Part model, mm, in its own coordinate system. Face numbers are marked on the shaded views. A direction names the side the tool comes from. Give positions to 0.01 mm unless a question says otherwise; leave off trailing zeros. Order: outer loops, then holes, each group sorted by start corner. A loop starts at its lowest first (then second) coordinate and runs counter-clockwise, first axis right, second up. Notation, with made-up numbers: (75, 21.25) - (114, 21.25) arc R11 cw to (114, 37.25) - close; hole circle Ø4 at (-21.5, 58). An arc over 180 degrees is marked (long way). One line per item, written item: value.
Autodesk Inventor part; units mm, degrees
ref_plane "YZ Plane" through (0, 0, 0) normal (1, 0, 0) x (0, 1, 0)
ref_plane "XZ Plane" through (0, 0, 0) normal (0, 1, 0) x (-1, 0, 0)
ref_plane "XY Plane" through (0, 0, 0) normal (0, 0, 1) x (1, 0, 0)
sketch "Эскиз1" plane through (0, 0, 0) normal (0, 0, 1) x (1, 0, 0)
  line L0 (-15, -15) -> (15, -15)
  line L1 (15, -15) -> (15, 15)
  line L2 (15, 15) -> (-15, 15)
  line L3 (-15, 15) -> (-15, -15)
  line L4 (-15, -15) -> (15, 15) construction
  line L5 (15, -15) -> (-15, 15) construction
  line L6 (15, 15) -> (20, 15)
  line L7 (20, 15) -> (20, -15)
  line L8 (20, -15) -> (15, -15)
  line L9 (15, -15) -> (15, 15)
  point P0 (0, 0)
  dimension "d0" = 30
  dimension "d1" = 30
  dimension "d2" = 5
extrude "Выдавливание1" add sketch "Эскиз1" along normal blind 5
sketch "Эскиз2" plane through (0, 0, 0) normal (0, 0, -1) x (-1, 0, 0)
  line L0 (-20, -15) -> (-20, 15)
  line L1 (15, -15) -> (-20, -15)
  line L2 (-20, 15) -> (-15, 15)
  line L3 (-15, 15) -> (-15, -15)
  line L4 (-15, -15) -> (-20, -15)
  line L5 (-20, -15) -> (-20, 15)
  point P0 (0, 0)
  dimension "d7" = 5
extrude "Выдавливание2" add sketch "Эскиз2" along normal blind 30
sketch "Эскиз3" plane through (0, 0, 5) normal (0, 0, 1) x (1, 0, 0)
  line L0 (-15, 15) -> (-15, -15)
  line L1 (-15, 0) -> (0, 0)
  circle A0 centre (0, 0) radius 4.1
  dimension "d10" = 15
  dimension "d11" = 8.2
sketch "Эскиз4" plane through (20, -15, 5) normal (1, 0, 0) x (0, 0, -1)
  line L0 (35, 30) -> (35, 0)
  line L1 (35, 15) -> (20, 15)
  circle A0 centre (20, 15) radius 4.1
  point P0 (5, 15)
  dimension "d12" = 15
  dimension "d13" = 8.2
sketch "Эскиз5" plane through (-15, 15, 5) normal (0, 1, 0) x (1, 0, 0)
  line L0 (30, 5) -> (30, 35)
  line L1 (30, 5) -> (50, 5)
  line L2 (50, 5) -> (50, -15)
  line L3 (50, -15) -> (30, -15)
  line L4 (30, -15) -> (30, 5)
  point P0 (15, 5)
  dimension "d18" = 20
  dimension "d19" = 20
extrude "Выдавливание5" add sketch "Эскиз5" against normal blind 5
chamfer "Фаска1" distance 15 angle 45 2 edges at (20, 12.5, 0) (15, 12.5, 5)
chamfer "Фаска2" distance 10 angle 45 2 edges at (17.5, 10, 5) (20, 10, 2.5)
extrude "Выдавливание6" cut sketch "Эскиз3" along normal blind 5 and the other way blind 16.25
extrude "Выдавливание7" cut sketch "Эскиз4" along normal blind 5 and the other way blind 11.5
sketch "Эскиз6" plane through (0, 0, 5) normal (0, 0, 1) x (1, 0, 0)
  circle A0 centre (0, 0) radius 7.5
  dimension "d38" = 15
extrude "Выдавливание8" cut sketch "Эскиз6" along normal blind 10.5
sketch "Эскиз7" plane through (20, -15, -30) normal (1, 0, 0) x (0, 0, -1)
  arc A0 (-19.1, 15) -> (-15, 19.1) centre (-15, 15) ccw
  circle A1 centre (-15, 15) radius 7.5
  point P0 (-30, 15)
  point P1 (-15, 10.9)
  dimension "d41" = 15
extrude "Выдавливание9" cut sketch "Эскиз7" along normal blind 10.5
sketch "Эскиз8" plane through (-15, 15, 5) normal (0, 1, 0) x (1, 0, 0)
  line L0 (35, 0) -> (45, -10)
  circle A0 centre (42.5, -7.5) radius 4.1
  point P0 (15, 5)
  point P1 (50, -15)
  dimension "d44" = 8.2
extrude "Выдавливание10" cut sketch "Эскиз8" against normal blind 17.25
sketch "Эскиз9" plane through (-15, 10, 5) normal (0, -1, 0) x (1, 0, 0)
  arc A0 (39.2504, 10) -> (39.6009, 4.6009) centre (42.5, 7.5) ccw
  circle A1 centre (42.5, 7.5) radius 7.5
  point P0 (15, -5)
  dimension "d47" = 15
extrude "Выдавливание11" cut sketch "Эскиз9" along normal blind 24
properties part number "КВ33.044.003 - крепеж дна блока управления" material "Пластик АБС"
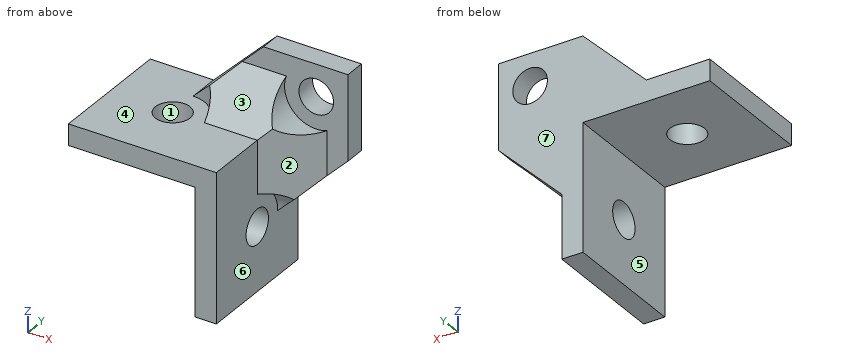
1) Cut at C-C, the plane z = -12.5. Give the cut face in (x, y).
Outcome:
outline: (15, -15) - (20, -15) - (20, -3.25) - (15, -3.25) - close; (15, 3.25) - (20, 3.25) - (20, 7.07) - (22.5, 7.07) - (22.5, 15) - (15, 15) - close
2) Drill centre lines: line 1 along X through (y, z) = (12.8, 12.5); line 2 along Z through (x, y) = (16.2, 0); line 3 along Y through (x, z) = (0, 2.65). Where is each one in solid material? Low to high. Write a range as from..to.
Outcome:
line 1: x = 7.5..23.4, 31.6..35
line 2: z = -30..-19.1, -10.9..5
line 3: y = -15..-4.1, 4.1..15
3) Mould opens along X. For the marked faces 1, 2 and 3 say: released by +X, released by -X, zero draft, split by the parting line, or undercut.
Outcome:
face 1: undercut
face 2: released by +X
face 3: zero draft
4) Cut at A-A, the plane x = 18.5. Give the cut face in (y, z), then the cut area to 3 significant figures.
Outcome:
outline: (-15, -30) - (15, -30) - (15, 20) - (10, 20) - (10, 15) - (0, 5) - (-15, 5) - close; hole circle Ø8.2 at (0, -15)
area: 1,120 mm^2
5) Cut at B-B, the plane z = 1.5. Give the cut face in (x, y), then the cut area to 3 significant figures.
Outcome:
outline: (-15, -15) - (20, -15) - (20, 0) - (30, 10) - (35, 10) - (35, 15) - (-15, 15) - close; hole circle Ø8.2 at (0, 0)
area: 1,120 mm^2
6) Cut at D-D, the plane x = 27.5. Give the cut face in (y, z).
Outcome:
outline: (7.5, -7.5) - (15, -7.5) - (15, 8.4) - (10, 8.4) - (10, 5) - (7.5, 5) - close; (10, 16.6) - (15, 16.6) - (15, 20) - (10, 20) - close
7) Pin check, flat tips, straight feed: pin 1 (12 mm diameter, centred on x = 26.5, z = -10.5, fed in from -Y); pin 2 (15 mm diameter, centred on x = -7.5, y = -4.5, fed in from -Z); pin 3 (1.5 mm diameter, centred on x = 5, y = -4, fed in from +Z); pin 4 (6.5 mm diameter, centred on x = 0, y = 0, fed in from +Z). Stop position of each tip, or through.
Outcome:
pin 1: stops at y = 1.25
pin 2: stops at z = 0
pin 3: stops at z = 5
pin 4: passes through
8) Which spindle directions (+Z, -Z, +X, -X, +Y, -Y) get a long thin tool onto all of the face, cutting with end or side? Do the marked faces 4, 5, 6 and 7. Say none if no direction does.
Outcome:
face 4: +Z, -X, -Y
face 5: -Z, -X, +Y, -Y
face 6: -Z, +X, -Y
face 7: +Z, -Z, +X, -X, +Y
